from build123d import *

# Parameters (mm, degrees)
SKETCH1_W               = 115
SKETCH1_H               = 115
BOSS_EXTRUDE1_DEPTH     = 35
SHELL2_T                = 5
SKETCH4_W               = 100
SKETCH4_H               = 90
CUT_EXTRUDE1_DEPTH      = 30
SKETCH5_W               = 95
SKETCH5_H               = 90
CUT_EXTRUDE2_DEPTH      = 30
FILLET1_R               = 10
CUT_EXTRUDE3_DEPTH      = 129.962203765
CUT_EXTRUDE3_DEPTH_BACK = 129.962203765
SKETCH9_W               = 25
SKETCH9_H               = 4


with BuildPart() as part:
    # Sketch1 → Boss-Extrude1 (new body)
    with BuildSketch(Plane.XY):
        Rectangle(SKETCH1_W, SKETCH1_H)
    extrude(amount=BOSS_EXTRUDE1_DEPTH)

    # Shell2 (no face opened: a closed hollow body)
    add(offset(amount=-SHELL2_T, mode=Mode.PRIVATE), mode=Mode.SUBTRACT)

    # Sketch4 → Cut-Extrude1 (cut)
    with BuildSketch(Plane.XY.offset(35)):
        with Locations((0, -5)):
            Rectangle(SKETCH4_W, SKETCH4_H)
    extrude(amount=-CUT_EXTRUDE1_DEPTH, mode=Mode.SUBTRACT)

    # Sketch5 → Cut-Extrude2 (cut)
    with BuildSketch(Plane(origin=(0, 0, 0), x_dir=(-1, 0, 0), z_dir=(0, 0, -1))):
        with Locations((0, 2.5)):
            Rectangle(SKETCH5_W, SKETCH5_H)
    extrude(amount=-CUT_EXTRUDE2_DEPTH, mode=Mode.SUBTRACT)

    # Fillet1
    fillet1_edges = [part.edges().sort_by_distance(p)[0] for p in [
        (-47.5, -42.5, 2.5),
        (47.5, -42.5, 2.5),
        (47.5, 47.5, 2.5),
        (-47.5, 47.5, 2.5),
    ]]
    fillet(fillet1_edges, radius=FILLET1_R)

    # Sketch9 → Cut-Extrude3 (cut, two sides: drawn at the far end of the back side and taken through both)
    with BuildSketch(Plane(origin=(-52.5, 0, 0), x_dir=(0, 0, -1), z_dir=(1, 0, 0)).offset(-CUT_EXTRUDE3_DEPTH_BACK)):
        with Locations((-17.5, -50.5)):
            Rectangle(SKETCH9_W, SKETCH9_H)
    extrude(amount=CUT_EXTRUDE3_DEPTH + CUT_EXTRUDE3_DEPTH_BACK, mode=Mode.SUBTRACT)


solid = part.part
Input: part model. Units: mm. Frame: model coordinates. A direction names the side the tool comes from. Coordinates: 2 decimals unless noted, no trailing zeros. Loops run counter-clockwise (first coordinate to the right, second up) from the corner with the lowest first, then second, coordinate; pieces in that order, holes last.
(1) Set-up query: faces 5 (the face through (-47.5, 2, 2)), 6 (the face through (1, 47.5, 2)), 7 (the face through (-52.5, 1, 17)). Return all of +Z, -Z, +X, -X, +Y, -Y with unobstructed straight access to the full face (end or side cutting, diameter ignored); none if empty.
(2) Section C-C on x = -18.5. Return the cut outline in (y, z).
(3) Material intervals for probe 1 along X at (y, z) = (18, 19.5); probe 2 along X at (y, z) = (5.5, 3.5), sorted ascending.
(4) Section D-D on y = -44. Return the cut outline in (x, z).
(5) Pull-direction query (Y, two-part tool) for faces 1 (the face through (-1, -57.5, 17)), 2 (the face through (-1, 57.5, 17)), 3 (the face through (50.3, 0.8, 35)), 4 (the face through (-44.49, -39.65, 2.54)); classes: released by +Y, released by -Y, zero draft, split by the parting line, or undercut.
(6) Section A-A on y = -25. Return the cut outline in (x, z), then the cut area to 3 significant figures.
(7) Section B-B on z = 15.5. Return the cut outline in (x, y), then the cut area to 3 significant figures.
Data:
1. face 5: +Z, -Z
1. face 6: -Z
1. face 7: none
2. outline: (-57.5, 0) - (-42.5, 0) - (-42.5, 5) - (-52.5, 5) - (-52.5, 30) - (-50, 30) - (-50, 35) - (-57.5, 35) - close; (40, 30) - (52.5, 30) - (52.5, 5) - (47.5, 5) - (47.5, 0) - (57.5, 0) - (57.5, 35) - (40, 35) - close
3. probe 1: x = -57.5 to -52.5, 52.5 to 57.5
3. probe 2: x = -57.5 to -47.5, 47.5 to 57.5
4. outline: (-57.5, 0) - (57.5, 0) - (57.5, 35) - (50, 35) - (50, 30) - (52.5, 30) - (52.5, 5) - (-52.5, 5) - (-52.5, 30) - (-50, 30) - (-50, 35) - (-57.5, 35) - close
5. face 1: released by -Y
5. face 2: released by +Y
5. face 3: zero draft
5. face 4: undercut
6. outline: (-57.5, 0) - (-47.5, 0) - (-47.5, 5) - (-52.5, 5) - (-52.5, 30) - (-50, 30) - (-50, 35) - (-57.5, 35) - close; (47.5, 0) - (57.5, 0) - (57.5, 35) - (50, 35) - (50, 30) - (52.5, 30) - (52.5, 5) - (47.5, 5) - close
6. area: 425 mm2
7. outline: (-57.5, -57.5) - (57.5, -57.5) - (57.5, -52.5) - (-57.5, -52.5) - close; (-57.5, -48.5) - (-52.5, -48.5) - (-52.5, 52.5) - (52.5, 52.5) - (52.5, -48.5) - (57.5, -48.5) - (57.5, 57.5) - (-57.5, 57.5) - close
7. area: 2,160 mm2
